from build123d import *

# Parameters (mm, degrees)
ESQUISSE1_R             = 10.85
ESQUISSE1_R_2           = 9
BOSS_EXTRU_1_DEPTH      = 7
ESQUISSE2_R             = 18
BOSS_EXTRU_2_DEPTH      = 2
ESQUISSE4_R             = 18
BOSS_EXTRU_3_DEPTH      = 4
BOSS_EXTRU_3_TAPER      = 74.5
ESQUISSE5_R             = 1.5
ENL_V_MAT_EXTRU_1_DEPTH = 4
ESQUISSE6_R             = 3.9
ENL_V_MAT_EXTRU_2_DEPTH = 4


with BuildPart() as part:
    # Esquisse1 → Boss.-Extru.1 (new body)
    with BuildSketch(Plane(origin=(0, 0, 0), x_dir=(1, 0, 0), z_dir=(0, 1, 0))):
        with Locations(Location((0, 0, 0), (0, 0, 270))):
            Circle(ESQUISSE1_R)
        with Locations(Location((0, 0, 0), (0, 0, 270))):
            Circle(ESQUISSE1_R_2, mode=Mode.SUBTRACT)
    extrude(amount=BOSS_EXTRU_1_DEPTH)

    # Esquisse2 → Boss.-Extru.2 (add)
    with BuildSketch(Plane(origin=(0, 7, 0), x_dir=(1, 0, 0), z_dir=(0, 1, 0))):
        with Locations(Location((0, 0, 0), (0, 0, 270))):
            Circle(ESQUISSE2_R)
    extrude(amount=BOSS_EXTRU_2_DEPTH)

    # Esquisse4 → Boss.-Extru.3 (add)
    with BuildSketch(Plane(origin=(0, 9, 0), x_dir=(1, 0, 0), z_dir=(0, 1, 0))):
        with Locations(Location((0, 0, 0), (0, 0, 270))):
            Circle(ESQUISSE4_R)
    extrude(amount=BOSS_EXTRU_3_DEPTH, taper=BOSS_EXTRU_3_TAPER)

    # Esquisse5 → Enlèv. mat.-Extru.1 (cut)
    with BuildSketch(Plane.XZ.offset(-7)):
        with Locations(Location((-12.898733794, 8.041309999, 0), (0, 0, 270))):
            Circle(ESQUISSE5_R)
        with Locations(Location((13.413345636, 7.149976143, 0), (0, 0, 270))):
            Circle(ESQUISSE5_R)
        with Locations(Location((-0.514611842, -15.191286142, 0), (0, 0, 270))):
            Circle(ESQUISSE5_R)
    extrude(amount=-ENL_V_MAT_EXTRU_1_DEPTH, mode=Mode.SUBTRACT)

    # Esquisse6 → Enlèv. mat.-Extru.2 (cut)
    with BuildSketch(Plane(origin=(0, 13, 0), x_dir=(1, 0, 0), z_dir=(0, 1, 0))):
        with Locations((-0.514611842, 15.191286142)):
            Circle(ESQUISSE6_R)
        with Locations((13.413345636, -7.149976143)):
            Circle(ESQUISSE6_R)
        with Locations((-12.898733794, -8.041309999)):
            Circle(ESQUISSE6_R)
    extrude(amount=-ENL_V_MAT_EXTRU_2_DEPTH, mode=Mode.SUBTRACT)


solid = part.part
Input: part model. Units: mm. Frame: model coordinates. A direction names the side the tool comes from. Coordinates: 2 decimals unless noted, no trailing zeros. Loops run counter-clockwise (first coordinate to the right, second up) from the corner with the lowest first, then second, coordinate; pieces in that order, holes last. Notation, with made-up numbers: (79.5, 33.5) -> (129.5, 33.5) arc R20 cw to (129.5, 67.5) -> close; hole circle Ø6 at (76, 30.5). An arc over 180 degrees is marked (long way). Write item = value, one per line. Start each with the question number.
Item 1: Cut plane B-B, the plane z = 0. Return loops of the section in (x, y).
Item 2: Reachability of faces 1 (the face through (-0.449, 7.986, -13.693)), 2 (the face through (10.03, 9.74, 5.21)), 3 (the face through (0, 7, 0)) from +Z, -Z, +X, -X, +Y, -Y: full face, straight path, thin tool, end or side. Return the list, or none.
Item 3: First-contact query: P1, Ø4, axis at x = -0.51, z = -15.19, coming from the -Y side; P2, Ø2.5, axis at x = 13.41, z = 7.15, coming from the -Y side; P3, Ø7, axis at x = 13.41, z = 7.15, coming from the +Y side; P4, Ø5.5, axis at x = 1, z = -16.5, coming from the +Y side. Flat tips, straight axial feed; report the tip coordinate or a pass-through.
Item 4: Material intervals for line 1 (X direction, y = 3.75, z = 0); line 2 (X direction, y = 5.25, z = -2.5); line 3 (Y direction, x = 6, z = 5.5), sorted ascending.
Item 5: Mould query, pull axis X, two halves, no side actions, for faces 4 (the face through (-11, 9, 8)), 5 (the face through (-9.52, 9.74, 6.09)), 6 (the face through (3.26, 3.45, 10.35)), 7 (the face through (0, 13, 0)). Classes: pulls with the +X half, pulls with the -X half, needs draft (parallel to the pull), parting line crosses it, or undercut.
Item 6: Cut plane A-A, the plane y = 1.5. Return loops of the section in (x, z).
Item 7: Cut plane C-C, the plane z = 7.5. Count the separate pieces of the cut face and the enclosed holes in it, plus the area to 3 significant figures.
Ans:
q1.outline = (-18, 7) -> (-10.85, 7) -> (-10.85, 0) -> (-9, 0) -> (-9, 7) -> (9, 7) -> (9, 0) -> (10.85, 0) -> (10.85, 7) -> (18, 7) -> (18, 9) -> (3.58, 13) -> (-3.58, 13) -> (-18, 9) -> close
q2.face_1 = +Y, -Y
q2.face_2 = +Y
q2.face_3 = -Y
q3.P1 = 7
q3.P2 = through
q3.P3 = 9
q3.P4 = 9.69
q4.line_1 = -10.85 to -9, 9 to 10.85
q4.line_2 = -10.56 to -8.65, 8.65 to 10.56
q4.line_3 = 7 to 11.73
q5.face_4 = undercut
q5.face_5 = undercut
q5.face_6 = parting line crosses it
q5.face_7 = needs draft
q6.outline = circle Ø21.7 at (0, 0); hole circle Ø18 at (0, 0)
q7.separate_pieces = 3
q7.enclosed_holes = 0
q7.area = 140 mm²
